Part model, mm, in its own coordinate system. A direction names the side the tool comes from. Round coordinates to 2 decimals unless told otherwise and drop trailing zeros. Return JSON: item names as keys, results as strings. Group by question number.
```python
from build123d import *

# Parameters (mm, degrees)
SKETCH1_R               = 3.695
SKETCH1_W               = 2.05
SKETCH1_H               = 32.2
SKETCH1_W_2             = 26.7
BOSS_EXTRUDE1_DEPTH     = 8
CUT_EXTRUDE1_DEPTH      = 58.637669713
CUT_EXTRUDE1_DEPTH_BACK = 58.637669713
SKETCH2_W               = 17.334925969
SKETCH2_H               = 2
SKETCH2_W_2             = 11.186287382
CUT_EXTRUDE2_DEPTH      = 59.676664498
CUT_EXTRUDE2_DEPTH_BACK = 59.676664498
SKETCH5_W               = 45.85613932
SKETCH5_H               = 2
SKETCH6_W               = 0.7
SKETCH6_H               = 11.18952338
SKETCH6_W_2             = 11.219404543
SKETCH6_H_2             = 0.7
SKETCH6_H_3             = 11.186287382
SKETCH6_W_3             = 11.186287383
BOSS_EXTRUDE2_DEPTH     = 4
SKETCH7_W               = 11.186287383
SKETCH7_H               = 0.6
BOSS_EXTRUDE3_DEPTH     = 1
CHAMFER1_SIZE           = 1
SKETCH8_W               = 11.219404543
SKETCH8_H               = 0.6
BOSS_EXTRUDE4_DEPTH     = 1
CHAMFER2_SIZE           = 1
SKETCH9_W               = 0.999620658
SKETCH9_H               = 4
CUT_EXTRUDE3_DEPTH      = 0.999620658
CUT_EXTRUDE4_REACH      = 64.753
SKETCH10_W              = 0.999620658
SKETCH10_H              = 4
CUT_EXTRUDE5_REACH      = 64.753
SKETCH11_W              = 0.999620658
SKETCH11_H              = 4
CUT_EXTRUDE6_REACH      = 65.709
SKETCH12_W              = 0.999620658
SKETCH12_H              = 4


with BuildPart() as part:
    # Sketch1 → Boss-Extrude1 (new body)
    with BuildSketch(Plane(origin=(0, 0, 0), x_dir=(1, 0, 0), z_dir=(0, 1, 0))):
        with BuildLine():
            ThreePointArc((-26.486246099, 27.414111587), (-32.658298898, 27.371294009), (-32.701116476, 21.19924121))
            Line((-32.701116476, 21.19924121), (-20.928398332, 4.665158012))
            Line((-20.928398332, 4.665158012), (-20.358176439, 3.864315241))
            Line((-20.358176439, 3.864315241), (-20.358176439, -7.321972141))
            Line((-20.358176439, -7.321972141), (-20.928398332, -8.122814912))
            Line((-20.928398332, -8.122814912), (-32.701116476, -24.65689811))
            ThreePointArc((-32.701116476, -24.65689811), (-32.658298898, -30.828950909), (-26.486246099, -30.871768487))
            Line((-26.486246099, -30.871768487), (-9.952162901, -19.099050343))
            Line((-9.952162901, -19.099050343), (-9.151320131, -18.52882845))
            Line((-9.151320131, -18.52882845), (2.034967252, -18.52882845))
            Line((2.034967252, -18.52882845), (2.835810023, -19.099050343))
            Line((2.835810023, -19.099050343), (19.369893221, -30.871768487))
            ThreePointArc((19.369893221, -30.871768487), (25.54194602, -30.828950909), (25.584763598, -24.65689811))
            Line((25.584763598, -24.65689811), (13.812045453, -8.122814912))
            Line((13.812045453, -8.122814912), (13.241823561, -7.321972141))
            Line((13.241823561, -7.321972141), (13.241823561, 3.864315241))
            Line((13.241823561, 3.864315241), (13.812045453, 4.665158012))
            Line((13.812045453, 4.665158012), (25.584763598, 21.19924121))
            ThreePointArc((25.584763598, 21.19924121), (25.54194602, 27.371294009), (19.369893221, 27.414111587))
            Line((19.369893221, 27.414111587), (2.835810023, 15.641393443))
            Line((2.835810023, 15.641393443), (2.034967252, 15.07117155))
            Line((2.034967252, 15.07117155), (-9.151320131, 15.07117155))
            Line((-9.151320131, 15.07117155), (-9.952162901, 15.641393443))
            Line((-9.952162901, 15.641393443), (-26.486246099, 27.414111587))
        make_face()
        with Locations(Location((-29.550564595, -27.721216605, 0), (0, 0, 270))):
            Circle(SKETCH1_R, mode=Mode.SUBTRACT)
        with BuildLine():
            Line((-20.358176439, -8.52882845), (-20.358176439, -18.52882845))
            Line((-20.358176439, -18.52882845), (-10.358176439, -18.52882845))
            Line((-10.358176439, -18.52882845), (-25.435304322, -29.264154677))
            ThreePointArc((-25.435304322, -29.264154677), (-26.442830291, -24.613482302), (-31.093502666, -23.605956333))
            Line((-31.093502666, -23.605956333), (-20.358176439, -8.52882845))
        make_face(mode=Mode.SUBTRACT)
        with Locations((-18.633176439, -1.72882845)):
            Rectangle(SKETCH1_W, SKETCH1_H, mode=Mode.SUBTRACT)
        with Locations((-3.558176439, -1.72882845)):
            Rectangle(SKETCH1_W_2, SKETCH1_H, mode=Mode.SUBTRACT)
        with Locations(Location((22.434211716, -27.721216605, 0), (0, 0, 270))):
            Circle(SKETCH1_R, mode=Mode.SUBTRACT)
        with BuildLine():
            ThreePointArc((23.977149788, -23.605956333), (19.326477413, -24.613482302), (18.318951444, -29.264154677))
            Line((18.318951444, -29.264154677), (3.241823561, -18.52882845))
            Line((3.241823561, -18.52882845), (13.241823561, -18.52882845))
            Line((13.241823561, -18.52882845), (13.241823561, -8.52882845))
            Line((13.241823561, -8.52882845), (23.977149788, -23.605956333))
        make_face(mode=Mode.SUBTRACT)
        with Locations((11.516823561, -1.72882845)):
            Rectangle(SKETCH1_W, SKETCH1_H, mode=Mode.SUBTRACT)
        with BuildLine():
            Line((-10.358176439, 15.07117155), (-20.358176439, 15.07117155))
            Line((-20.358176439, 15.07117155), (-20.358176439, 5.07117155))
            Line((-20.358176439, 5.07117155), (-31.093502666, 20.148299433))
            ThreePointArc((-31.093502666, 20.148299433), (-26.442830291, 21.155825402), (-25.435304322, 25.806497777))
            Line((-25.435304322, 25.806497777), (-10.358176439, 15.07117155))
        make_face(mode=Mode.SUBTRACT)
        with Locations(Location((-29.550564595, 24.263559705, 0), (0, 0, 270))):
            Circle(SKETCH1_R, mode=Mode.SUBTRACT)
        with BuildLine():
            Line((13.241823561, 5.07117155), (13.241823561, 15.07117155))
            Line((13.241823561, 15.07117155), (3.241823561, 15.07117155))
            Line((3.241823561, 15.07117155), (18.318951444, 25.806497777))
            ThreePointArc((18.318951444, 25.806497777), (19.326477413, 21.155825402), (23.977149788, 20.148299433))
            Line((23.977149788, 20.148299433), (13.241823561, 5.07117155))
        make_face(mode=Mode.SUBTRACT)
        with Locations(Location((22.434211716, 24.263559705, 0), (0, 0, 270))):
            Circle(SKETCH1_R, mode=Mode.SUBTRACT)
    extrude(amount=BOSS_EXTRUDE1_DEPTH)

    # Sketch2 → Cut-Extrude1 (cut, two sides: drawn at the far end of the back side and taken through both)
    with BuildSketch(Plane.ZY.offset(20.358176439).offset(-CUT_EXTRUDE1_DEPTH_BACK)):
        with Locations((-12.531778226, 5)):
            Rectangle(SKETCH2_W, SKETCH2_H)
        with Locations((1.72882845, 5)):
            Rectangle(SKETCH2_W_2, SKETCH2_H)
        with Locations((15.989435126, 5)):
            Rectangle(SKETCH2_W, SKETCH2_H)
        with Locations((-12.531778226, 3)):
            Rectangle(SKETCH2_W, SKETCH2_H)
        with Locations((1.72882845, 3)):
            Rectangle(SKETCH2_W_2, SKETCH2_H)
        with Locations((15.989435126, 3)):
            Rectangle(SKETCH2_W, SKETCH2_H)
    extrude(amount=CUT_EXTRUDE1_DEPTH + CUT_EXTRUDE1_DEPTH_BACK, mode=Mode.SUBTRACT)

    # Sketch5 → Cut-Extrude2 (cut, two sides: drawn at the far end of the back side and taken through both)
    with BuildSketch(Plane(origin=(0, 0, -15.07117155), x_dir=(-1, 0, 0), z_dir=(0, 0, -1)).offset(-CUT_EXTRUDE2_DEPTH_BACK)):
        Polygon((-19.369893221, 6), (-19.369893221, 4), (26.486246099, 4), (26.486246099, 6), (9.151320131, 6), (-2.034967252, 6), align=None)
        with Locations((3.558176439, 3)):
            Rectangle(SKETCH5_W, SKETCH5_H)
    extrude(amount=CUT_EXTRUDE2_DEPTH + CUT_EXTRUDE2_DEPTH_BACK, mode=Mode.SUBTRACT)

    # Sketch6 → Boss-Extrude2 (add)
    with BuildSketch(Plane(origin=(0, 2, 0), x_dir=(1, 0, 0), z_dir=(0, 1, 0))):
        with Locations((-20.008176439, -1.730446449)):
            Rectangle(SKETCH6_W, SKETCH6_H)
        with Locations((-3.54161786, -18.17882845)):
            Rectangle(SKETCH6_W_2, SKETCH6_H_2)
        with Locations((12.891823561, -1.72882845)):
            Rectangle(SKETCH6_W, SKETCH6_H_3)
        with Locations((-3.55817644, 14.72117155)):
            Rectangle(SKETCH6_W_3, SKETCH6_H_2)
    extrude(amount=BOSS_EXTRUDE2_DEPTH)

    # Sketch7 → Boss-Extrude3 (add)
    with BuildSketch(Plane.XY.offset(-14.37117155)):
        with Locations((-3.55817644, 5.7)):
            Rectangle(SKETCH7_W, SKETCH7_H)
    extrude(amount=BOSS_EXTRUDE3_DEPTH)

    # Chamfer1
    chamfer1_edges = [part.edges().sort_by_distance(p)[0] for p in [
        (-3.558176439, 5.4, -14.37117155),
    ]]
    chamfer(chamfer1_edges, length=CHAMFER1_SIZE - 0.0001)  # a hair under: the kernel refuses the full size

    # Sketch8 → Boss-Extrude4 (add)
    with BuildSketch(Plane(origin=(0, 0, 17.82882845), x_dir=(-1, 0, 0), z_dir=(0, 0, -1))):
        with Locations((3.54161786, 5.7)):
            Rectangle(SKETCH8_W, SKETCH8_H)
    extrude(amount=BOSS_EXTRUDE4_DEPTH)

    # Chamfer2
    chamfer2_edges = [part.edges().sort_by_distance(p)[0] for p in [
        (-3.541617859, 5.4, 17.82882845),
    ]]
    chamfer(chamfer2_edges, length=CHAMFER2_SIZE - 0.0001)  # a hair under: the kernel refuses the full size

    # Sketch9 → Cut-Extrude3 (cut)
    with BuildSketch(Plane(origin=(0, 0, 24.65689811), x_dir=(-1, 0, 0), z_dir=(0, 0, -1))):
        with Locations((-19.86970355, 4)):
            Rectangle(SKETCH9_W, SKETCH9_H)
    extrude(amount=-CUT_EXTRUDE3_DEPTH, mode=Mode.SUBTRACT)

    # Sketch10 → Cut-Extrude4 (cut, up to next)
    with BuildSketch(Plane(origin=(-26.486246099, 0, 0), x_dir=(0, 0, -1), z_dir=(1, 0, 0)), mode=Mode.PRIVATE) as cut_extrude4_sk1:
        with Locations((-25.156708439, 4)):
            Rectangle(SKETCH10_W, SKETCH10_H)
    cut_extrude4_tool1 = extrude(cut_extrude4_sk1.sketch, amount=-CUT_EXTRUDE4_REACH, mode=Mode.PRIVATE) & part.part
    add(cut_extrude4_tool1.solids().sort_by_distance((-26.486246, 4, 25.156708))[0], mode=Mode.SUBTRACT)

    # Sketch11 → Cut-Extrude5 (cut, up to next)
    with BuildSketch(Plane(origin=(-26.486246099, 0, 0), x_dir=(0, 0, -1), z_dir=(1, 0, 0)), mode=Mode.PRIVATE) as cut_extrude5_sk1:
        with Locations((21.699051539, 4)):
            Rectangle(SKETCH11_W, SKETCH11_H)
    cut_extrude5_tool1 = extrude(cut_extrude5_sk1.sketch, amount=-CUT_EXTRUDE5_REACH, mode=Mode.PRIVATE) & part.part
    add(cut_extrude5_tool1.solids().sort_by_distance((-26.486246, 4, -21.699052))[0], mode=Mode.SUBTRACT)

    # Sketch12 → Cut-Extrude6 (cut, up to next)
    with BuildSketch(Plane.XY.offset(-21.19924121), mode=Mode.PRIVATE) as cut_extrude6_sk1:
        with Locations((19.86970355, 4)):
            Rectangle(SKETCH12_W, SKETCH12_H)
    cut_extrude6_tool1 = extrude(cut_extrude6_sk1.sketch, amount=-CUT_EXTRUDE6_REACH, mode=Mode.PRIVATE) & part.part
    add(cut_extrude6_tool1.solids().sort_by_distance((19.869704, 4, -21.199241))[0], mode=Mode.SUBTRACT)


solid = part.part
```
Item 1: Two-plate mould, pull along X, no slides. Class faces 1 (the face through (-9.151, 4, 18)), 2 (the face through (19.277, 6.986, -21.206)), 3 (the face through (13.242, 7, 14)): released by +X, released by -X, zero draft, split by the parting line, or undercut.
Item 2: Which spindle directions (+Z, -Z, +X, -X, +Y, -Y) get a long thin tool onto all of the face, cutting with end or side? Do faces 4 (the face through (-20.358, 4, 2)), 5 (the face through (-3, 4, -15.071)), 6 (the face through (10, 2, 2)), 7 (the face through (10.886, 6.986, 23.972)). Say none if no direction does.
Item 3: Flat gauge pins, fed straight in: P1, Ø9.5, axis at x = -29.55, z = 27.72, coming from the +Y side; P2, Ø2, axis at x = -16.5, y = 7.5, coming from the +Z side; P3, Ø1, axis at y = 6.5, z = 18, coming from the +X side; P4, Ø4, axis at x = -3.5, y = 5.5, coming from the +Z side. Where does each tip first touch, or does it go through?
Item 4: Wall check: L1, parallel to X at y = 7.25, z = 4; L2, parallel to Z at x = 22, y = 6.5; L3, parallel to Z at x = -13, y = 6.5. Give the ranges that are in metal, low to high.
Item 5: Cut at B-B (y = 3.25). State how many separate pieces and enclosed holes the cut face has, then the cut area to 3 significant figures.
Checks:
{
 "1": {"face 1": "released by -X", "face 2": "undercut", "face 3": "undercut"},
 "2": {"face 4": "-X, +Y, -Y", "face 5": "-Z, +Y, -Y", "face 6": "none", "face 7": "+Y, -Y"},
 "3": {"P1": "stops at y = 8", "P2": "stops at z = 24.47", "P3": "stops at x = 21.2", "P4": "stops at z = 18.53"},
 "4": {"L1": "x = -20.36 to -19.66, -17.61 to -16.91, 9.79 to 10.49, 12.54 to 13.24", "L2": "z = -28.64 to -27.93, -20.59 to -19.89, -17.37 to -16.16, 19.62 to 20.83, 23.35 to 24.05, 31.39 to 32.09", "L3": "z = -17.81 to -16.95, -15.07 to -14.37, 17.83 to 18.53, 20.41 to 21.27"},
 "5": {"separate pieces": "8", "enclosed holes": "0", "area": "68.7 mm2"}
}
